from build123d import *

# Parameters (mm, degrees)
SKETCH1_W           = 42
SKETCH1_H           = 42
BOSS_EXTRUDE1_DEPTH = 11
CHAMFER1_SIZE       = 3
SKETCH4_R           = 11.25
BOSS_EXTRUDE2_DEPTH = 0.5
CUT_EXTRUDE4_REACH  = 33.67
SKETCH8_R           = 1.5


with BuildPart() as part:
    # Sketch1 → Boss-Extrude1 (new body)
    with BuildSketch(Plane.XY):
        Rectangle(SKETCH1_W, SKETCH1_H)
    extrude(amount=BOSS_EXTRUDE1_DEPTH)

    # Chamfer1
    chamfer1_edges = [part.edges().sort_by_distance(p)[0] for p in [
        (-21, 21, 5.5),
        (21, 21, 5.5),
        (21, -21, 5.5),
        (-21, -21, 5.5),
    ]]
    chamfer(chamfer1_edges, length=CHAMFER1_SIZE)

    # Sketch4 → Boss-Extrude2 (add)
    with BuildSketch(Plane(origin=(0, 0, 0), x_dir=(-1, 0, 0), z_dir=(0, 0, -1))):
        Circle(SKETCH4_R)
    extrude(amount=-BOSS_EXTRUDE2_DEPTH)

    # Sketch8 → Cut-Extrude4 (cut, up to next)
    with BuildSketch(Plane(origin=(0, 0, 0), x_dir=(-1, 0, 0), z_dir=(0, 0, -1)), mode=Mode.PRIVATE) as cut_extrude4_sk1:
        with Locations((15.5, 15.5)):
            Circle(SKETCH8_R)
    cut_extrude4_tool1 = extrude(cut_extrude4_sk1.sketch, amount=-CUT_EXTRUDE4_REACH, mode=Mode.PRIVATE) & part.part
    # Sketch8 → Cut-Extrude4 (cut, up to next)
    with BuildSketch(Plane(origin=(0, 0, 0), x_dir=(-1, 0, 0), z_dir=(0, 0, -1)), mode=Mode.PRIVATE) as cut_extrude4_sk2:
        with Locations((-15.5, 15.5)):
            Circle(SKETCH8_R)
    cut_extrude4_tool2 = extrude(cut_extrude4_sk2.sketch, amount=-CUT_EXTRUDE4_REACH, mode=Mode.PRIVATE) & part.part
    # Sketch8 → Cut-Extrude4 (cut, up to next)
    with BuildSketch(Plane(origin=(0, 0, 0), x_dir=(-1, 0, 0), z_dir=(0, 0, -1)), mode=Mode.PRIVATE) as cut_extrude4_sk3:
        with Locations((-15.5, -15.5)):
            Circle(SKETCH8_R)
    cut_extrude4_tool3 = extrude(cut_extrude4_sk3.sketch, amount=-CUT_EXTRUDE4_REACH, mode=Mode.PRIVATE) & part.part
    # Sketch8 → Cut-Extrude4 (cut, up to next)
    with BuildSketch(Plane(origin=(0, 0, 0), x_dir=(-1, 0, 0), z_dir=(0, 0, -1)), mode=Mode.PRIVATE) as cut_extrude4_sk4:
        with Locations((15.5, -15.5)):
            Circle(SKETCH8_R)
    cut_extrude4_tool4 = extrude(cut_extrude4_sk4.sketch, amount=-CUT_EXTRUDE4_REACH, mode=Mode.PRIVATE) & part.part
    add(cut_extrude4_tool1.solids().sort_by_distance((-15.5, 15.5, 0))[0], mode=Mode.SUBTRACT)
    add(cut_extrude4_tool2.solids().sort_by_distance((15.5, 15.5, 0))[0], mode=Mode.SUBTRACT)
    add(cut_extrude4_tool3.solids().sort_by_distance((15.5, -15.5, 0))[0], mode=Mode.SUBTRACT)
    add(cut_extrude4_tool4.solids().sort_by_distance((-15.5, -15.5, 0))[0], mode=Mode.SUBTRACT)


solid = part.part
Verification items for the finished model (mm, model axes). Give positions to 0.01 mm unless a question says otherwise; leave off trailing zeros. Loops run counter-clockwise (first coordinate to the right, second up) from the corner with the lowest first, then second, coordinate; pieces in that order, holes last.
1. Release check for a two-part mould opening along Y. For faces 1 (the flat face through (0, 21, 5)), 2 (the cylindrical face through (17, 15.57, 5.42)), 3 (the flat face through (0, -21, 5)), 4 (the flat face through (0, 0, 0)) record: +Y half, -Y half, draft (parallel to the pull), parting line (faces both ways), or undercut.
Derived:
face 1: +Y half
face 2: undercut
face 3: -Y half
face 4: draft
2. Go/stop test with flat-tipped pins: P1, Ø5, axis at x = 15.5, y = -15.5, coming from the -Z side; P2, Ø2.5, axis at x = 15.5, y = 15.5, coming from the -Z side. Record where each tip stops, or that it passes through.
Derived:
P1: stops at z = 0
P2: passes through
3. Cross-section at A-A on y = 15.5. Record the cut outline in (x, z), and give its area (3 significant figures).
Derived:
outline: (-21, 0) - (-17, 0) - (-17, 11) - (-21, 11) - close; (-14, 0) - (14, 0) - (14, 11) - (-14, 11) - close; (17, 0) - (21, 0) - (21, 11) - (17, 11) - close
area: 396 mm2
4. Material ranges on probe 1 along Y at (x, z) = (15.5, 4.5); probe 2 along X at (y, z) = (16.5, 2.5); probe 3 along Y at (x, z) = (-16, 8), recorded low to high.
Derived:
probe 1: y = -21 to -17, -14 to 14, 17 to 21
probe 2: x = -21 to -16.62, -14.38 to 14.38, 16.62 to 21
probe 3: y = -21 to -16.91, -14.09 to 14.09, 16.91 to 21
5. Cross-section at C-C on z = 3.75. Record the cut outline in (x, y).
Derived:
outline: (-21, -18) - (-18, -21) - (18, -21) - (21, -18) - (21, 18) - (18, 21) - (-18, 21) - (-21, 18) - close; hole circle Ø3 at (-15.5, -15.5); hole circle Ø3 at (-15.5, 15.5); hole circle Ø3 at (15.5, -15.5); hole circle Ø3 at (15.5, 15.5)
